Build history of the part. All positions in model axes, mm. Face numbers are marked on the shaded views. A direction names the side the tool comes from. Coordinates: 2 decimals unless noted, no trailing zeros. Loops run counter-clockwise (first coordinate to the right, second up) from the corner with the lowest first, then second, coordinate; pieces in that order, holes last.
Item 1: Cut at B-B (y = 0). List the corners of the cut face in (x, z) (3 decimals), and give its area (3 significant figures).
Item 2: Flat gauge pins, fed straight in: pin 1 (1.5 mm diameter, centred on y = -2.5, z = 9, fed in from +X); pin 2 (1.5 mm diameter, centred on y = -1, z = 13, fed in from -X); pin 3 (4 mm diameter, centred on y = -5.5, z = 10.5, fed in from -X). Where does each tip first touch, or does it go through?
Item 3: Cut at C-C (x = 25.5). List the corners of the cut face in (y, z) (3 decimals), and give its area (3 significant figures).
Item 4: 3-axis set-ups, long thin cutter, end or side, ignore diameter. For the marked faces 3 and 4: which of +Z, -Z, +X, -X, +Y, -Y reach the whole face in a straight line?
Item 5: Drill centre lines: line 1 along X through (y, z) = (1, 14); line 2 along Y through (x, z) = (33, 11) (3 decimals); line 3 along Z through (x, y) = (14, -4). Where is each one in solid material? Low to high.
Item 6: Mould opens along X. For the marked faces 1 and 2 say: released by +X, released by -X, zero draft, split by the parting line, or undercut.
Item 7: Cut at A-A (z = 7). List the corners of the cut face in (x, y) (3 decimals).
from build123d import *

# Parameters (mm, degrees)
ESBO_O1_R                  = 1.5
RESSALTO_EXTRUS_O1_DEPTH   = 15
CORTE_EXTRUS_O1_DEPTH      = 40.769162048
CORTE_EXTRUS_O1_DEPTH_BACK = 40.769162048
ESBO_O2_W                  = 23.1
ESBO_O2_H                  = 12.2


with BuildPart() as part:
    # Esboço1 → Ressalto-extrusão1 (new body)
    with BuildSketch(Plane.XY):
        with BuildLine():
            Line((0, 3.175), (33, 3.175))
            ThreePointArc((33, 3.175), (36.162475296, -0.281735692), (32.438751392, -3.125))
            Line((32.438751392, -3.125), (32.438751392, -6.925))
            Line((32.438751392, -6.925), (0.561248608, -6.925))
            Line((0.561248608, -6.925), (0.561248608, -3.125))
            ThreePointArc((0.561248608, -3.125), (-3.162475296, -0.281735692), (0, 3.175))
        make_face()
        Circle(ESBO_O1_R, mode=Mode.SUBTRACT)
        with Locations((33, 0)):
            Circle(ESBO_O1_R, mode=Mode.SUBTRACT)
    extrude(amount=RESSALTO_EXTRUS_O1_DEPTH)

    # Esboço2 → Corte-extrusão1 (cut, two sides: drawn at the far end of the back side and taken through both)
    with BuildSketch(Plane(origin=(0, 0, 0), x_dir=(1, 0, 0), z_dir=(0, 1, 0)).offset(-CORTE_EXTRUS_O1_DEPTH_BACK)):
        with Locations((16.5, -8.9)):
            Rectangle(ESBO_O2_W, ESBO_O2_H)
    extrude(amount=CORTE_EXTRUS_O1_DEPTH + CORTE_EXTRUS_O1_DEPTH_BACK, mode=Mode.SUBTRACT)


solid = part.part
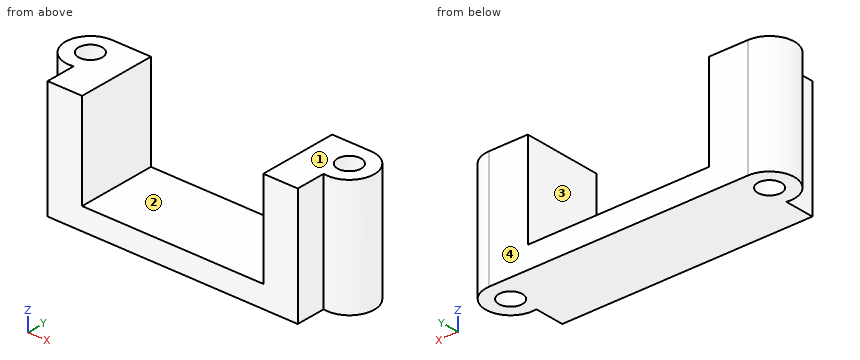
Filled sheet:
1. outline: (-3.175, 0) - (-1.5, 0) - (-1.5, 15) - (-3.175, 15) - close; (1.5, 0) - (31.5, 0) - (31.5, 15) - (28.05, 15) - (28.05, 2.8) - (4.95, 2.8) - (4.95, 15) - (1.5, 15) - close; (34.5, 0) - (36.175, 0) - (36.175, 15) - (34.5, 15) - close
1. area: 218 mm2
2. pin 1: stops at x = 35.65
2. pin 2: stops at x = -3.17
2. pin 3: stops at x = 0.56
3. outline: (-6.925, 0) - (3.175, 0) - (3.175, 2.8) - (-6.925, 2.8) - close
3. area: 28.3 mm2
4. face 3: +Z, +Y, -Y
4. face 4: +Z, -Z, +X, -X, +Y
5. line 1: x = -3.01 to -1.12, 1.12 to 4.95, 28.05 to 31.88, 34.12 to 36.01
5. line 2: y = -3.175 to -1.5, 1.5 to 3.175
5. line 3: z = 0 to 2.8
6. face 1: zero draft
6. face 2: undercut
7. outline: (0, 3.175) arc R3.175 ccw (long way) to (0.561, -3.125) - (0.561, -6.925) - (4.95, -6.925) - (4.95, 3.175) - close; (28.05, -6.925) - (32.439, -6.925) - (32.439, -3.125) arc R3.175 ccw (long way) to (33, 3.175) - (28.05, 3.175) - close; hole circle Ø3 at (0, 0); hole circle Ø3 at (33, 0)
